Check sheet for the drawn part. Datum: minimum x, y, z corner. Units: mm. A direction names the side the tool comes from. Coordinates: 2 decimals unless noted, no trailing zeros. Loops run counter-clockwise (first coordinate to the right, second up) from the corner with the lowest first, then second, coordinate; pieces in that order, holes last.
Q1. Mould release check, pull along X, two halves, no side actions. Record for the marked faces 1, 2 and 3: +X half, -X half, draft (parallel to the pull), parting line (faces both ways), or undercut.
Q2. Access from +Z, -Z, +X, -X, +Y, -Y to the whole of each face (thin tool, end or side, straight path). Record for the marked faces 4, 5, 6, 7 and 8.
Q3. Sectioned sample at B-B (z = 13). Enter the section's corners in (x, y).
Q4. Sectioned sample at D-D (x = 6). Enter the section's corners in (y, z), then the cut area to 3 significant figures.
Q5. Sectioned sample at C-C (y = 21). Enter the section's corners in (x, z).
Q6. Material ranges on probe 1 along X at (y, z) = (6.5, 6); probe 2 along Y at (x, z) = (13, 3); probe 3 along Y at (x, z) = (17.5, 13), recorded low to high.
Q7. Sectioned sample at A-A (x = 31). Enter the section's corners in (y, z), then the cut area to 3 significant figures.
Q8. Go/stop test with flat-tipped pins: P1, Ø2, axis at y = 26, z = 2, coming from the -X side; P2, Ø6, axis at x = 6, y = 59.5, coming from the +Z side; P3, Ø2, axis at x = 12, y = 20, coming from the +Z side; P4, Ø2, axis at y = 26.5, z = 3, coming from the +X side. Record where each tip stops, or that it passes through.
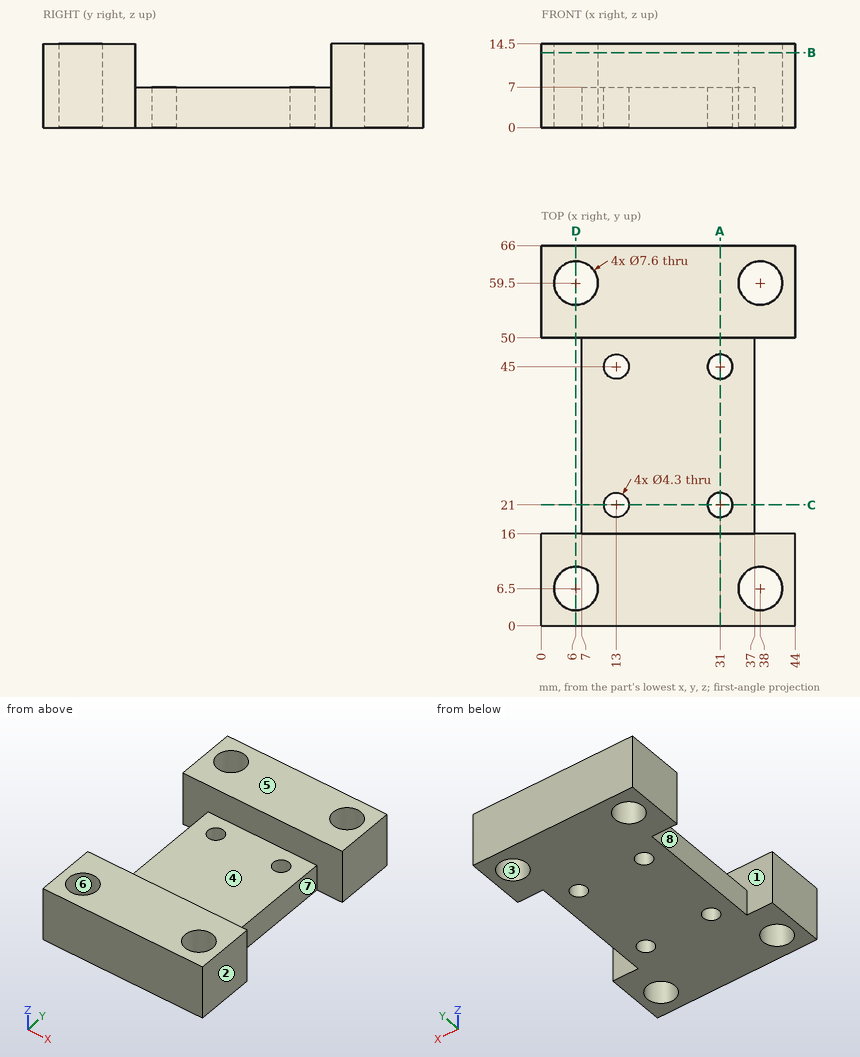
Geometry check:
1. face 1: draft
1. face 2: +X half
1. face 3: undercut
2. face 4: +Z, +X, -X
2. face 5: +Z, +X, -X, +Y, -Y
2. face 6: +Z, -Z
2. face 7: +Z, -Z, +X
2. face 8: +Z, -Z, -X
3. outline: (0, 0) - (44, 0) - (44, 16) - (0, 16) - close; (0, 50) - (44, 50) - (44, 66) - (0, 66) - close; hole circle Ø7.6 at (6, 6.5); hole circle Ø7.6 at (6, 59.5); hole circle Ø7.6 at (38, 6.5); hole circle Ø7.6 at (38, 59.5)
4. outline: (0, 0) - (2.7, 0) - (2.7, 14.5) - (0, 14.5) - close; (10.3, 0) - (16, 0) - (16, 14.5) - (10.3, 14.5) - close; (50, 0) - (55.7, 0) - (55.7, 14.5) - (50, 14.5) - close; (63.3, 0) - (66, 0) - (66, 14.5) - (63.3, 14.5) - close
4. area: 244 mm2
5. outline: (7, 0) - (10.85, 0) - (10.85, 7) - (7, 7) - close; (15.15, 0) - (28.85, 0) - (28.85, 7) - (15.15, 7) - close; (33.15, 0) - (37, 0) - (37, 7) - (33.15, 7) - close
6. probe 1: x = 0 to 2.2, 9.8 to 34.2, 41.8 to 44
6. probe 2: y = 0 to 18.85, 23.15 to 42.85, 47.15 to 66
6. probe 3: y = 0 to 16, 50 to 66
7. outline: (0, 0) - (18.85, 0) - (18.85, 7) - (16, 7) - (16, 14.5) - (0, 14.5) - close; (23.15, 0) - (42.85, 0) - (42.85, 7) - (23.15, 7) - close; (47.15, 0) - (66, 0) - (66, 14.5) - (50, 14.5) - (50, 7) - (47.15, 7) - close
7. area: 642 mm2
8. P1: stops at x = 7
8. P2: passes through
8. P3: stops at z = 7
8. P4: stops at x = 37
